from build123d import *

# Parameters (mm, degrees)
F1_DEPTH = 3.175
F2_R     = 3.81
F3_DEPTH = 25.4
F6_DEPTH = 6.35


with BuildPart() as f1:
    # F0 (on Front) → F1 (new body)
    with BuildSketch(Plane.XZ):
        with BuildLine():
            Line((-17.960512, -10.480528), (-11.973675, -27.413861))
            ThreePointArc((-11.973675, -27.413861), (0, -35.880528), (11.973675, -27.413861))
            Line((11.973675, -27.413861), (17.960512, -10.480528))
            ThreePointArc((17.960512, -10.480528), (0, 14.919472), (-17.960512, -10.480528))
        make_face()
    extrude(amount=F1_DEPTH)

    # F2 (on face) → F3 (cut)
    with BuildSketch(Plane.XZ.offset(3.175)):
        with Locations((0, 6.029472)):
            Circle(F2_R)
        with Locations((0, -26.990528)):
            Circle(F2_R)
    extrude(amount=-F3_DEPTH, mode=Mode.SUBTRACT)

    # F5 (on offset) → F6 (join)
    with BuildSketch(Plane.YZ.offset(3.175)):
        with BuildLine():
            Line((-15.357632, -5.726944), (-6.861671, -20.32))
            Line((-6.861671, -20.32), (-3.175, -20.32))
            Line((-3.175, -20.32), (-3.175, -12.826101))
            Line((-3.175, -12.826101), (-5.018335, -12.826101))
            Line((-5.018335, -12.826101), (-8.419373, -2.702977))
            ThreePointArc((-8.419373, -2.702977), (-13.58725, -0.317314), (-15.357632, -5.726944))
        make_face()
    extrude(amount=-F6_DEPTH)


solid = f1.part
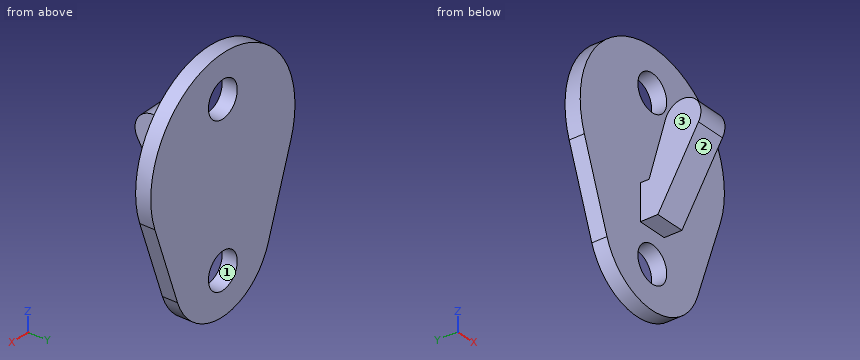
Can you work these out from the model? Positions are in its coordinate system, mm. Face numbers are marked on the shaded views. Give positions to 0.01 mm unless a question says otherwise; leave off trailing zeros. Loops run counter-clockwise (first coordinate to the right, second up) from the corner with the lowest first, then second, coordinate; pieces in that order, holes last. Notation, with made-up numbers: M 37.5,23 L 71.5,23 A17 ccw 71.5,50 Z; hole C -0.5,79 d8. An arc over 180 degrees is marked long. One line per item, written item: value. Start each with the question number.
1) Thinking about a two-plate mould opening in X: for the marked faces 1, 2 and 3, which applies, +X half, -X half, draft (parallel to the pull), parting line (faces both ways), or undercut?
2) If we section it at A-A, the plane x = 0: Write out the boundary of the cut face in (y, z) (3 decimals), and give its area (3 significant figures).
3) If we section it at C-C, the plane z = -3.81: Write out the boundary of the cut face in (x, y) (3 decimals), and give its area (3 significant figures).
4) If we section it at B-B, the plane z = -26: Write out the boundary of the cut face in (x, y) (3 decimals), and give its area (3 significant figures).
5) If I drill on line 1 (Z direction, x = 0, y = -2.5); line 2 (Y direction, x = -10, z = 7.5) (3 decimals); line 3 (Y direction, x = 3, z = -11.5) (3 decimals), over which ranges is the centre line in solid material (lowest first)? Write a range as [from, to].
6) If we section it at D-D, the plane x = -6: Write out the boundary of the cut face in (y, z) (3 decimals), and give its area (3 significant figures).
7) I'm going to push flat-ended pins straight in: pin 1 (3 mm diameter, centred on x = -1, y = -6, fed in from -Z); pin 2 (8 mm diameter, centred on x = 13.5, z = 4.5, fed in from -Y) (3 decimals); pin 3 (8 mm diameter, centred on y = -5, z = -9.5, fed in from -X); pin 4 (1.5 mm diameter, centred on y = -10, z = -18, fed in from +X). Where does each tip first touch, or does it pass through?
Completed:
1. face 1: undercut
1. face 2: draft
1. face 3: -X half
2. outline: M -15.358,-5.727 L -6.862,-20.32 L -3.175,-20.32 L -3.175,-23.181 L 0,-23.181 L 0,2.219 L -3.175,2.219 L -3.175,-12.826 L -5.018,-12.826 L -8.419,-2.703 A3.81 ccw long Z; M -3.175,-35.881 L 0,-35.881 L 0,-30.801 L -3.175,-30.801 Z; M -3.175,9.839 L 0,9.839 L 0,14.919 L -3.175,14.919 Z
2. area: 245 mm^2
3. outline: M -19.047,-3.175 L 19.047,-3.175 L 19.047,0 L -19.047,0 Z; M -3.175,-15.875 L 3.175,-15.875 L 3.175,-8.047 L -3.175,-8.047 Z
3. area: 171 mm^2
4. outline: M -12.474,-3.175 L -3.679,-3.175 L -3.679,0 L -12.474,0 Z; M 3.679,-3.175 L 12.474,-3.175 L 12.474,0 L 3.679,0 Z
4. area: 55.8 mm^2
5. line 1: z = [-35.88, -30.8], [-23.18, 2.22], [9.84, 14.92]
5. line 2: y = [-3.175, 0]
5. line 3: y = [-11.997, -5.464], [-3.175, 0]
6. outline: M -3.175,-34.374 L 0,-34.374 L 0,13.95 L -3.175,13.95 Z
6. area: 153 mm^2
7. pin 1: stops at z = -20.32
7. pin 2: stops at y = -3.175
7. pin 3: stops at x = -18.96
7. pin 4: passes through
